from build123d import *

# Parameters (mm, degrees)
SKETCH_3_R          = 12.55
SKETCH_3_R_2        = 6.55
EXTRUDE_1_DEPTH     = 3
CUT_EXTRUDE_3_DEPTH = 337.61902384
EXTRUDE_2_DEPTH     = 3
CHAMFER_1_SIZE      = 4
CHAMFER_1_SIZE2     = 3.120824035
CHAMFER_2_SIZE      = 4
CHAMFER_2_SIZE2     = 3.866160824
CHAMFER_3_SIZE      = 4
CHAMFER_3_SIZE2     = 23.911485469
SKETCH_8_R          = 1
CUT_EXTRUDE_4_DEPTH = 336.947679111
SKETCH_9_R          = 1.1
SKETCH_9_R_2        = 1.6
CUT_EXTRUDE_5_DEPTH = 336.947679111
FILLET_1_R          = 50
CUT_EXTRUDE_6_DEPTH = 335.374368924
FILLET_2_R          = 1
FILLET_3_R          = 1
EXTRUDE_3_DEPTH     = 3


with BuildPart() as part:
    # 草图3 → 凸台-拉伸1 (new body)
    # profile 1 of 4: a face of its own
    with BuildSketch(Plane(origin=(0, 0, 0), x_dir=(1, 0, 0), z_dir=(0, 1, 0))):
        with BuildLine():
            Line((121.265604443, 289.597455686), (128.868463655, 240.178870804))
            Line((128.868463655, 240.178870804), (141.647697325, 191.053787979))
            Line((141.647697325, 191.053787979), (108.429878461, 83.756455888))
            ThreePointArc((108.429878461, 83.756455888), (92.967297732, 44.045236663), (72.033938301, 6.925608458))
            ThreePointArc((72.033938301, 6.925608458), (86.116173784, 12.017728037), (95.05, 0))
            ThreePointArc((95.05, 0), (94.935972216, -1.687926254), (94.59596095, -3.34517992))
            ThreePointArc((94.59596095, -3.34517992), (96.273603044, 2.110037129), (98.259734457, 7.460659342))
            Line((98.259734457, 7.460659342), (171.571212245, 188.912934219))
            Line((171.571212245, 188.912934219), (140.881048659, 285.694335372))
            Line((140.881048659, 285.694335372), (121.265604443, 289.597455686))
        make_face()
    # profile 2 of 4: a face of its own
    with BuildSketch(Plane(origin=(0, 0, 0), x_dir=(1, 0, 0), z_dir=(0, 1, 0))):
        with Locations((82.5, 0)):
            Circle(SKETCH_3_R)
        with Locations(Location((82.5, 0, 0), (0, 0, 270))):
            Circle(SKETCH_3_R_2, mode=Mode.SUBTRACT)
    # profile 3 of 4: a face of its own
    with BuildSketch(Plane(origin=(0, 0, 0), x_dir=(1, 0, 0), z_dir=(0, 1, 0))):
        with BuildLine():
            ThreePointArc((94.59596095, -3.34517992), (82.5, -12.55), (70.40403905, -3.34517992))
            ThreePointArc((70.40403905, -3.34517992), (74.021880086, -30), (70.40403905, -56.65482008))
            ThreePointArc((70.40403905, -56.65482008), (82.5, -47.45), (94.59596095, -56.65482008))
            ThreePointArc((94.59596095, -56.65482008), (90.978119914, -30), (94.59596095, -3.34517992))
        make_face()
    # profile 4 of 4: a face of its own
    with BuildSketch(Plane(origin=(0, 0, 0), x_dir=(1, 0, 0), z_dir=(0, 1, 0))):
        with Locations((82.5, -60)):
            Circle(SKETCH_3_R)
        with Locations(Location((82.5, -60, 0), (0, 0, 270))):
            Circle(SKETCH_3_R_2, mode=Mode.SUBTRACT)
    extrude(amount=EXTRUDE_1_DEPTH)

    # 草图7 → 切除-拉伸3 (cut, through all)
    with BuildSketch(Plane(origin=(0, 3, 0), x_dir=(1, 0, 0), z_dir=(0, 1, 0))):
        with BuildLine():
            ThreePointArc((78.002512198, -34.493479197), (80.195428175, -33.349158141), (81.33105467, -31.151726999))
            ThreePointArc((81.33105467, -31.151726999), (81.29055467, -30.45576741), (81.33105467, -29.75980782))
            ThreePointArc((81.33105467, -29.75980782), (79.648864591, -27.101907795), (76.578597142, -26.418055622))
            ThreePointArc((76.578597142, -26.418055622), (74.734518785, -25.952185157), (73.857268025, -24.264556235))
            ThreePointArc((73.857268025, -24.264556235), (74.006073686, -31.777928612), (73.590239535, -39.281260509))
            Line((73.590239535, -39.281260509), (78.002512198, -34.493479197))
        make_face()
    extrude(amount=-CUT_EXTRUDE_3_DEPTH, mode=Mode.SUBTRACT)

    # 草图7<3> → 凸台-拉伸2 (add)
    with BuildSketch(Plane(origin=(0, 3, 0), x_dir=(1, 0, 0), z_dir=(0, 1, 0))):
        with BuildLine():
            ThreePointArc((91.066651947, -25.793033303), (90.979085958, -30.43955416), (91.10749612, -35.085125677))
            ThreePointArc((91.10749612, -35.085125677), (91.947297407, -34.239250868), (92.603316411, -33.24405769))
            ThreePointArc((92.603316411, -33.24405769), (93.116212163, -31.891634666), (93.29055467, -30.45576741))
            ThreePointArc((93.29055467, -30.45576741), (92.937299887, -28.427401453), (91.919131852, -26.637878821))
            ThreePointArc((91.919131852, -26.637878821), (91.514069696, -26.194086893), (91.066651947, -25.793033303))
        make_face()
        with BuildLine():
            ThreePointArc((92.603316411, -33.24405769), (91.947297407, -34.239250868), (91.10749612, -35.085125677))
            ThreePointArc((91.10749612, -35.085125677), (91.236559388, -37.184782804), (91.409760465, -39.281260509))
            ThreePointArc((91.409760465, -39.281260509), (91.568630527, -36.176084637), (92.603316411, -33.24405769))
        make_face()
        with BuildLine():
            ThreePointArc((91.142731975, -24.264556235), (91.101768, -25.028649229), (91.066651947, -25.793033303))
            ThreePointArc((91.066651947, -25.793033303), (91.514069696, -26.194086893), (91.919131852, -26.637878821))
            ThreePointArc((91.919131852, -26.637878821), (91.306680236, -25.524578384), (91.142731975, -24.264556235))
        make_face()
    extrude(amount=-EXTRUDE_2_DEPTH)

    # 倒角1
    chamfer_1_edges = [part.edges().sort_by_distance(p)[0] for p in [
        (121.265604443, 1.5, -289.597455686),
    ]]
    chamfer_1_side = [part.faces().sort_by_distance(p)[0] for p in [
        (131.073326551, 1.5, -287.645895529),
    ]]
    chamfer(chamfer_1_edges, length=CHAMFER_1_SIZE, length2=CHAMFER_1_SIZE2, reference=chamfer_1_side[0])

    # 倒角2
    chamfer_2_edges = [part.edges().sort_by_distance(p)[0] for p in [
        (140.881048659, 1.5, -285.694335372),
    ]]
    chamfer_2_side = [part.faces().sort_by_distance(p)[0] for p in [
        (156.226130452, 1.5, -237.303634796),
    ]]
    chamfer(chamfer_2_edges, length=CHAMFER_2_SIZE, length2=CHAMFER_2_SIZE2, reference=chamfer_2_side[0])

    # 倒角3
    chamfer_3_edges = [part.edges().sort_by_distance(p)[0] for p in [
        (128.868463655, 1.5, -240.178870804),
    ]]
    chamfer_3_side = [part.faces().sort_by_distance(p)[0] for p in [
        (125.304305907, 1.5, -263.34589617),
    ]]
    chamfer(chamfer_3_edges, length=CHAMFER_3_SIZE, length2=CHAMFER_3_SIZE2, reference=chamfer_3_side[0])

    # 草图8 → 切除-拉伸4 (cut, through all)
    with BuildSketch(Plane(origin=(0, 3, 0), x_dir=(1, 0, 0), z_dir=(0, 1, 0))):
        with Locations((129.481912621, 280.519443616)):
            Circle(SKETCH_8_R)
        with Locations((135.464623107, 279.32899192)):
            Circle(SKETCH_8_R)
        with Locations((128.818382167, 277.184818099)):
            Circle(SKETCH_8_R)
        with Locations((134.801092653, 275.994366404)):
            Circle(SKETCH_8_R)
        with Locations((147.653970306, 192.328419252)):
            Circle(SKETCH_8_R)
        with Locations((147.411340213, 188.937087561)):
            Circle(SKETCH_8_R)
        with Locations((161.718022318, 191.322217985)):
            Circle(SKETCH_8_R)
        with Locations((161.475392225, 187.930886294)):
            Circle(SKETCH_8_R)
        with Locations((112.339085524, 71.25713446)):
            Circle(SKETCH_8_R)
        with Locations((115.047221748, 69.201411183)):
            Circle(SKETCH_8_R)
        with Locations((120.86429088, 82.487934683)):
            Circle(SKETCH_8_R)
        with Locations((123.572427104, 80.432211406)):
            Circle(SKETCH_8_R)
        Polygon((128.50114041, 280.714599632), (136.445395318, 279.133835905), (135.781864864, 275.799210388), (127.837609957, 277.379974115), align=None)
        Polygon((146.656519808, 192.399781044), (162.715472815, 191.250856193), (162.472842723, 187.859524502), (146.413889715, 189.008449353), align=None)
        Polygon((111.734461031, 70.460623806), (121.468915373, 83.284445337), (124.177051597, 81.22872206), (114.442597255, 68.404900529), align=None)
    extrude(amount=-CUT_EXTRUDE_4_DEPTH, mode=Mode.SUBTRACT)

    # 草图9 → 切除-拉伸5 (cut, through all)
    with BuildSketch(Plane(origin=(0, 3, 0), x_dir=(1, 0, 0), z_dir=(0, 1, 0))):
        with Locations(Location((133.980578042, 235.236844896, 0), (0, 0, 270))):
            Circle(SKETCH_9_R)
        with Locations(Location((138.710717702, 215.804249115, 0), (0, 0, 270))):
            Circle(SKETCH_9_R)
        with Locations(Location((138.598734412, 171.061193721, 0), (0, 0, 270))):
            Circle(SKETCH_9_R)
        with Locations(Location((132.68396468, 151.955814923, 0), (0, 0, 270))):
            Circle(SKETCH_9_R)
        with Locations(Location((126.769194947, 132.850436126, 0), (0, 0, 270))):
            Circle(SKETCH_9_R)
        with Locations(Location((125.973199927, 118, 0), (0, 0, 270))):
            Circle(SKETCH_9_R_2)
        with Locations(Location((115.368060475, 89.937016958, 0), (0, 0, 270))):
            Circle(SKETCH_9_R_2)
        with Locations(Location((128.154092345, 101.140471292, 0), (0, 0, 270))):
            Circle(SKETCH_9_R_2)
    extrude(amount=-CUT_EXTRUDE_5_DEPTH, mode=Mode.SUBTRACT)

    # 圆角1
    fillet_1_edges = [part.edges().sort_by_distance(p)[0] for p in [
        (141.647697325, 1.5, -191.053787979),
        (171.571212245, 1.5, -188.912934219),
    ]]
    fillet(fillet_1_edges, radius=FILLET_1_R)

    # 草图11 → 切除-拉伸6 (cut, through all)
    with BuildSketch(Plane(origin=(0, 3, 0), x_dir=(1, 0, 0), z_dir=(0, 1, 0))):
        Polygon((141.594357666, 256.978870067), (150.289401614, 200.461084402), (159.730803103, 199.785606942), align=None)
        Polygon((146.804308515, 180.659302195), (159.248540878, 179.768989619), (139.564574089, 131.049462198), (131.621693467, 131.617729191), align=None)
    extrude(amount=-CUT_EXTRUDE_6_DEPTH, mode=Mode.SUBTRACT)

    # 圆角2
    fillet_2_edges = [part.edges().sort_by_distance(p)[0] for p in [
        (159.730803103, 1.5, -199.785606942),
        (150.289401614, 1.5, -200.461084402),
        (131.621693467, 1.5, -131.617729191),
        (146.804308515, 1.5, -180.659302195),
        (159.248540878, 1.5, -179.768989619),
        (139.564574089, 1.5, -131.049462198),
        (73.590239535, 1.5, 39.281260509),
        (78.002512198, 1.5, 34.493479197),
    ]]
    fillet(fillet_2_edges, radius=FILLET_2_R)

    # 圆角3
    fillet_3_edges = [part.edges().sort_by_distance(p)[0] for p in [
        (141.594357666, 1.5, -256.978870067),
    ]]
    fillet(fillet_3_edges, radius=FILLET_3_R)

    # 草图12 → 凸台-拉伸3 (add)
    with BuildSketch(Plane(origin=(0, 3, 0), x_dir=(1, 0, 0), z_dir=(0, 1, 0))):
        with BuildLine():
            Line((98.259734457, 7.460659342), (117.34519382, 54.698828901))
            ThreePointArc((117.34519382, 54.698828901), (100.675476378, -1.577194053), (95.05, -60))
            ThreePointArc((95.05, -60), (94.935972216, -58.312073746), (94.59596095, -56.65482008))
            ThreePointArc((94.59596095, -56.65482008), (92.618516623, -48.038526559), (91.409760465, -39.281260509))
            ThreePointArc((91.409760465, -39.281260509), (91.568630527, -36.176084637), (92.603316411, -33.24405769))
            ThreePointArc((92.603316411, -33.24405769), (93.258632644, -29.837669281), (91.919131852, -26.637878821))
            ThreePointArc((91.919131852, -26.637878821), (91.306680236, -25.524578384), (91.142731975, -24.264556235))
            ThreePointArc((91.142731975, -24.264556235), (93.403219258, -8.110761503), (98.259734457, 7.460659342))
        make_face()
        with BuildLine():
            ThreePointArc((81.33105467, -29.75980782), (79.648864591, -27.101907795), (76.578597142, -26.418055622))
            ThreePointArc((76.578597142, -26.418055622), (76.037227153, -26.449216759), (75.503392909, -26.353961938))
            ThreePointArc((75.503392909, -26.353961938), (78.962149718, -29.908542384), (77.787287008, -34.727021234))
            ThreePointArc((77.787287008, -34.727021234), (78.012719423, -34.54448268), (78.281056834, -34.43432311))
            ThreePointArc((78.281056834, -34.43432311), (80.294153345, -33.246537017), (81.33105467, -31.151726999))
            ThreePointArc((81.33105467, -31.151726999), (81.29055467, -30.45576741), (81.33105467, -29.75980782))
        make_face()
    extrude(amount=-EXTRUDE_3_DEPTH)


solid = part.part
Read the model definition and answer for the solid it produces. Units are mm, in the model's axes. A direction names the side the tool comes from. Give positions to 0.01 mm unless a question says otherwise; leave off trailing zeros. Write each loop counter-clockwise with the first axis right and the second up, starting at its lowest first coordinate (ties: lowest second). Pieces come first, ordered by that corner, then holes. Notation, with made-up numbers: (58.5, 39.25) - (113.5, 39.25) arc R22 cw to (113.5, 61.25) - close; hole circle Ø7 at (18, 63). An arc over 180 degrees is marked (long way). Answer in a Markdown table with one row per item. Add a question column.
Item 1: Determine the mould class of faces 1 (the face through (140.755, 1.479, -112.639)), 2 (the face through (154.28, 1.48, -243.44)), 3 (the face through (139.18, 1.52, -156.03)), 4 (the face through (116.55, 1.521, -76.805)) for opening direction Z: pulls with the +Z half, pulls with the -Z half, needs draft (parallel to the pull), parting line crosses it, or undercut.
Item 2: Section C-C, the plane z = 0 is taken. Write down the section's boundary in (x, y).
Item 3: Flat-ended cylindrical pins translate along their axes: P1, Ø2.5, axis at x = 128.15, z = -101.14, coming from the +Y side; P2, Ø1.5, axis at y = 0.5, z = -180.5, coming from the -X side; P3, Ø1.5, axis at y = 1.5, z = -173.5, coming from the +X side. Find the tip coordinate at first contact, or state that the pin passes through.
Item 4: Section B-B, the plane x = 82.5 is taken. Write down the section's boundary in (y, z).
Item 5: Section A-A, the plane z = -166 is taken. Write down the section's boundary in (x, y), and give its area (3 significant figures).
Item 6: Find the intervals of material crossed by L1, parallel to X at y = 1.4, z = -118; L2, parallel to X at y = 1.65, z = -215.5; L3, parallel to Z at x = 78, y = 1.8, in increasing order.
Item 7: Section D-D, the plane y = 2.3 is taken. Count the separate pieces of the cut face and the enclosed holes in it, and give its area (3 significant figures).
Item 8: A tool of negligible diameter and unlimited length cuts with its end or side. For faces 5 (the face through (131.62, 1.48, -230.4)), 6 (the face through (119.36, 1.52, -74.88)), 7 (the face through (123, 0, -109)), from which of +Z, -Z, +X, -X, +Y, -Y can it reach the whole face along a straight path? Write none if from no direction.
Recorded:
| question | item | result |
|---|---|---|
| 1 | face 1 | pulls with the +Z half |
| 1 | face 2 | pulls with the -Z half |
| 1 | face 3 | undercut |
| 1 | face 4 | undercut |
| 2 | outline | (69.95, 0) - (75.95, 0) - (75.95, 3) - (69.95, 3) - close; (89.05, 0) - (100.99, 0) - (100.99, 3) - (89.05, 3) - close |
| 3 | P1 | passes through |
| 3 | P2 | stops at x = 138.09 |
| 3 | P3 | stops at x = 165.6 |
| 4 | outline | (0, -23.95) - (3, -23.95) - (3, -6.55) - (0, -6.55) - close; (0, 6.55) - (3, 6.55) - (3, 53.45) - (0, 53.45) - close; (0, 66.55) - (3, 66.55) - (3, 72.55) - (0, 72.55) - close |
| 5 | outline | (133.89, 0) - (142.27, 0) - (142.27, 3) - (133.89, 3) - close; (153.69, 0) - (162.31, 0) - (162.31, 3) - (153.69, 3) - close |
| 5 | area | 51.0 mm2 |
| 6 | L1 | x = 119.03 to 124.37, 127.57 to 142.92 |
| 6 | L2 | x = 135.29 to 137.65, 139.77 to 147.98, 154.75 to 163.14 |
| 6 | L3 | z = -16.32 to -4.76, 4.76 to 28.03, 34.48 to 55.24, 64.76 to 71.72 |
| 7 | separate pieces | 1 |
| 7 | enclosed holes | 15 |
| 7 | area | 7,510 mm2 |
| 8 | face 5 | -X, +Y, -Y |
| 8 | face 6 | +Y, -Y |
| 8 | face 7 | +Z, -Z, +X, -X, -Y |
